```python
from build123d import *

# Parameters (mm, degrees)
F0_R     = 12.7
F1_DEPTH = 35.56
F2_R     = 8.636
F3_DEPTH = 9.525
F4_R     = 2.794
F5_DEPTH = 254
F6_R     = 8.636
F6_R_2   = 2.794
F8_DEPTH = 9.4488


with BuildPart() as f1:
    # F0 (on Top) → F1 (new body)
    with BuildSketch(Plane.XY):
        Circle(F0_R)
    extrude(amount=F1_DEPTH)

    # F2 (on face) → F3 (cut)
    with BuildSketch(Plane.XY.offset(35.56)):
        Circle(F2_R)
    extrude(amount=-F3_DEPTH, mode=Mode.SUBTRACT)

    # F4 (on face) → F5 (cut)
    with BuildSketch(Plane.XY.offset(26.035)):
        Circle(F4_R)
    extrude(amount=-F5_DEPTH, mode=Mode.SUBTRACT)

    # F6 (on face) → F8 (cut)
    with BuildSketch(Plane(origin=(0, 0, 0), x_dir=(1, 0, 0), z_dir=(0, 0, -1))):
        Circle(F6_R)
        Circle(F6_R_2, mode=Mode.SUBTRACT)
    extrude(amount=-F8_DEPTH, mode=Mode.SUBTRACT)


solid = f1.part
```
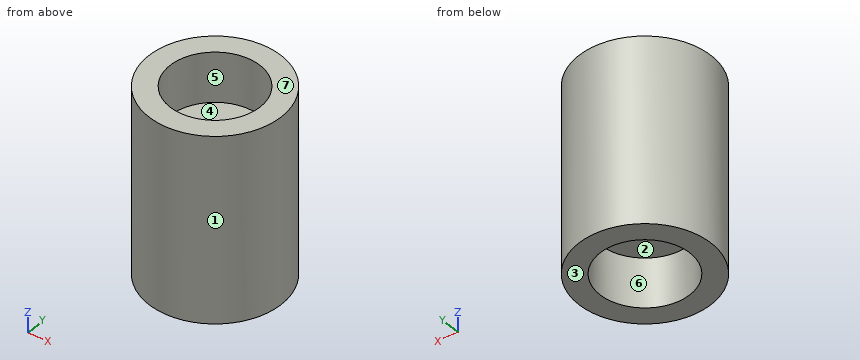
Build history of the part. All positions in model axes, mm. Face numbers are marked on the shaded views. A direction names the side the tool comes from. Round coordinates to 2 decimals unless told otherwise and drop trailing zeros. Loops run counter-clockwise (first coordinate to the right, second up) from the corner with the lowest first, then second, coordinate; pieces in that order, holes last.
Item 1: Drill centre lines: line 1 along Y through (x, z) = (0, 7); line 2 along X through (y, z) = (-0.25, 4.5); line 3 along Y through (x, z) = (0, 19). Where is each one in solid material? Low to high.
Item 2: Saw through at D-D (x = 5.75). List the corners of the cut face in (y, z) (3 decimals).
Item 3: Two-plate mould, pull along Y, no slides. Class the marked faces 1, 2, 3 and 4: released by +Y, released by -Y, zero draft, split by the parting line, or undercut.
Item 4: Saw through at C-C (z = 24). List the corners of the cut face in (x, y).
Item 5: Pin check, flat tips, straight feed: P1, Ø1.5, axis at x = 9.5, z = 16.5, coming from the -Y side; P2, Ø1, axis at y = 7.5, z = 30, coming from the +X side; P3, Ø6, axis at x = -6, y = -3.5, coming from the -Z side; P4, Ø1.5, axis at x = 3.5, z = 17, coming from the -Y side. Stop position of each tip, or through.
Item 6: Which spindle directions (+Z, -Z, +X, -X, +Y, -Y) get a long thin tool onto all of the face, cutting with end or side? Do the marked faces 5, 6 and 7. Say none if no direction does.
Item 7: Saw through at A-A (y = 0). List the corners of the cut face in (x, z) (3 decimals).
Worked answers:
1. line 1: y = -12.7 to -8.64, 8.64 to 12.7
1. line 2: x = -12.7 to -8.63, 8.63 to 12.7
1. line 3: y = -12.7 to -2.79, 2.79 to 12.7
2. outline: (-11.324, 0) - (-6.443, 0) - (-6.443, 9.449) - (6.443, 9.449) - (6.443, 0) - (11.324, 0) - (11.324, 35.56) - (6.443, 35.56) - (6.443, 26.035) - (-6.443, 26.035) - (-6.443, 35.56) - (-11.324, 35.56) - close
3. face 1: split by the parting line
3. face 2: undercut
3. face 3: zero draft
3. face 4: undercut
4. outline: circle Ø25.4 at (0, 0); hole circle Ø5.59 at (0, 0)
5. P1: stops at y = -9.2
5. P2: stops at x = 10.6
5. P3: stops at z = 0
5. P4: stops at y = -12.4
6. face 5: +Z
6. face 6: -Z
6. face 7: +Z, +X, -X, +Y, -Y
7. outline: (-12.7, 0) - (-8.636, 0) - (-8.636, 9.449) - (-2.794, 9.449) - (-2.794, 26.035) - (-8.636, 26.035) - (-8.636, 35.56) - (-12.7, 35.56) - close; (2.794, 9.449) - (8.636, 9.449) - (8.636, 0) - (12.7, 0) - (12.7, 35.56) - (8.636, 35.56) - (8.636, 26.035) - (2.794, 26.035) - close
